from build123d import *

# Parameters (mm, degrees)
F0_W     = 70
F0_H     = 75
F1_DEPTH = 125
F3_START = -20
F2_W     = 20
F2_H     = 75
F3_DEPTH = 105.001
F5_START = -55
F4_W     = 10
F4_H     = 75
F5_DEPTH = 25.5
F7_START = -30
F6_W     = 70
F6_H     = 25
F7_DEPTH = 70
F9_START = -20
F8_W     = 5
F8_H     = 75
F9_DEPTH = 60.5


with BuildPart() as f1:
    # F0 (on Right) → F1 (new body)
    with BuildSketch(Plane.YZ):
        with Locations((35, 37.5)):
            Rectangle(F0_W, F0_H)
    extrude(amount=F1_DEPTH)

    # F2 (on face) → F3 (cut)
    with BuildSketch(Plane.YZ.offset(125).offset(F3_START)):
        with Locations((10, 37.5)):
            Rectangle(F2_W, F2_H)
    extrude(amount=-F3_DEPTH, mode=Mode.SUBTRACT)

    # F4 (on face) → F5 (cut)
    with BuildSketch(Plane.YZ.offset(125).offset(F5_START)):
        with Locations((25, 37.5)):
            Rectangle(F4_W, F4_H)
    extrude(amount=-F5_DEPTH, mode=Mode.SUBTRACT)

    # F6 (on face) → F7 (cut)
    with BuildSketch(Plane.YZ.offset(125).offset(F7_START)):
        with Locations((35, 62.5)):
            Rectangle(F6_W, F6_H)
    extrude(amount=-F7_DEPTH, mode=Mode.SUBTRACT)

    # F8 (on face) → F9 (cut)
    with BuildSketch(Plane.YZ.offset(125).offset(F9_START)):
        with Locations((22.5, 37.5)):
            Rectangle(F8_W, F8_H)
    extrude(amount=-F9_DEPTH, mode=Mode.SUBTRACT)


solid = f1.part
Check sheet for the modelled part. Datum: model origin and axes. Units: mm. A direction names the side the tool comes from. Coordinates: 2 decimals unless noted, no trailing zeros. Loops run counter-clockwise (first coordinate to the right, second up) from the corner with the lowest first, then second, coordinate; pieces in that order, holes last. Notation, with made-up numbers: (8, 13.25) -> (12, 13.25) arc R20 cw to (12, 30.25) -> close; hole circle Ø4 at (71, 20.5). An arc over 180 degrees is marked (long way). Answer in a Markdown table with one row per item.
1. Sectioned sample at A-A, the plane z = 57.5. Record the boundary of the cut face in (x, y).
Check values:
| item | result |
|---|---|
| outline | (0, 20) -> (25, 20) -> (25, 70) -> (0, 70) -> close; (95, 25) -> (105, 25) -> (105, 0) -> (125, 0) -> (125, 70) -> (95, 70) -> close |
2. Sectioned sample at B-B, the plane y = 44. Record the boundary of the cut face in (x, z).
Check values:
| item | result |
|---|---|
| outline | (0, 0) -> (125, 0) -> (125, 75) -> (95, 75) -> (95, 50) -> (25, 50) -> (25, 75) -> (0, 75) -> close |
3. Material ranges on line 1 along X through (y, z) = (26.5, 42.5); line 2 along X through (y, z) = (21, 41); line 3 along Z through (x, y) = (72.5, 43.5), recorded low to high. Write a range as [from, to].
Check values:
| item | result |
|---|---|
| line 1 | x = [0, 44.5], [70, 125] |
| line 2 | x = [0, 44.5], [105, 125] |
| line 3 | z = [0, 50] |
4. Access from +Z, -Z, +X, -X, +Y, -Y to the whole of each face (thin tool, end or side, straight path). Record for faces 1 (the face through (88, 25, 29)), 2 (the face through (23, 20, 29)), 3 (the face through (25, 45, 63)).
Check values:
| item | result |
|---|---|
| face 1 | +Z, -Z, -Y |
| face 2 | +Z, -Z, -X, -Y |
| face 3 | +Z, +Y, -Y |
5. Release check for a two-part mould opening along X. For faces 4 (the face through (0, 45, 38)), 5 (the face through (115, 0, 37)), 6 (the face through (60, 50, 50)) record: released by +X, released by -X, zero draft, split by the parting line, or undercut.
Check values:
| item | result |
|---|---|
| face 4 | released by -X |
| face 5 | zero draft |
| face 6 | undercut |
6. Sectioned sample at C-C, the plane z = 27. Record the boundary of the cut face in (x, y).
Check values:
| item | result |
|---|---|
| outline | (0, 20) -> (44.5, 20) -> (44.5, 30) -> (70, 30) -> (70, 25) -> (105, 25) -> (105, 0) -> (125, 0) -> (125, 70) -> (0, 70) -> close |
7. Go/stop test with flat-tipped pins: pin 1 (7.5 mm diameter, centred on y = 10, z = 35.5, fed in from -X); pin 2 (1 mm diameter, centred on x = 65.5, y = 34, fed in from +Z); pin 3 (13 mm diameter, centred on x = 52, z = 37.5, fed in from -Y). Record where each tip stops, or that it passes through.
Check values:
| item | result |
|---|---|
| pin 1 | stops at x = 105 |
| pin 2 | stops at z = 50 |
| pin 3 | stops at y = 30 |
8. Sectioned sample at D-D, the plane x = 31. Record the boundary of the cut face in (y, z).
Check values:
| item | result |
|---|---|
| outline | (20, 0) -> (70, 0) -> (70, 50) -> (20, 50) -> close |
